Build history of the part. All positions in model axes, mm. A direction names the side the tool comes from. Give positions to 0.01 mm unless a question says otherwise; leave off trailing zeros. Write each loop counter-clockwise with the first axis right and the second up, starting at its lowest first coordinate (ties: lowest second). Pieces come first, ordered by that corner, then holes. Notation, with made-up numbers: (25, 58.25) -> (72, 58.25) arc R21 ccw to (72, 89.25) -> close; hole circle Ø8 at (42.25, 78.5). An arc over 180 degrees is marked (long way). Put each result on its own line as item: value.
from build123d import *

# Parameters (mm, degrees)
SKETCH_1_W                         = 406.5
SKETCH_1_H                         = 22
SM_BASE_FLANGE_1_DEPTH             = 2
SM_EDGE_FLANGE_1_STRIP_W           = 10
SM_EDGE_FLANGE_1_STRIP_H           = 2
SM_EDGE_FLANGE_1_STRIP_CUT_DEPTH   = 406.5
SM_EDGE_FLANGE_1_STRIP_2_W         = 10
SM_EDGE_FLANGE_1_STRIP_2_H         = 2
SM_EDGE_FLANGE_1_STRIP_CUT_2_DEPTH = 406.5
SM_EDGE_FLANGE_1_DEPTH             = 406.5
SM_EDGE_FLANGE_1_BEND_DEPTH        = 406.5
SM_EDGE_FLANGE_2_STRIP_W           = 10
SM_EDGE_FLANGE_2_STRIP_H           = 2
SM_EDGE_FLANGE_2_STRIP_CUT_DEPTH   = 16
SM_EDGE_FLANGE_2_STRIP_2_W         = 10
SM_EDGE_FLANGE_2_STRIP_2_H         = 2
SM_EDGE_FLANGE_2_STRIP_CUT_2_DEPTH = 16
SM_EDGE_FLANGE_2_DEPTH             = 16
SM_EDGE_FLANGE_2_BEND_DEPTH        = 16
SKETCH_18_W                        = 9
SKETCH_18_H                        = 9
CUT_EXTRUDE_1_DEPTH                = 10
PATTERN_LINEAR_1_COUNT             = 19
PATTERN_LINEAR_1_PITCH             = 20
FILLET_1_R                         = 5
SKETCH_19_R                        = 3.5
CUT_EXTRUDE_2_DEPTH                = 408.140332072


# Sheet-metal steps are written as plain solids
with BuildPart() as part:
    # Sketch 1 → 基体-法兰1 (new body)
    with BuildSketch(Plane.XY):
        Rectangle(SKETCH_1_W, SKETCH_1_H)
    extrude(amount=-SM_BASE_FLANGE_1_DEPTH)

    # 边线-法兰1 strip (across the edge) → 边线-法兰1 strip cut (cut)
    with BuildSketch(Plane(origin=(203.25, -11, -2), x_dir=(0, 1, 0), z_dir=(-1, 0, 0))):
        with Locations((-2, -1)):
            Rectangle(SM_EDGE_FLANGE_1_STRIP_W, SM_EDGE_FLANGE_1_STRIP_H)
    extrude(amount=SM_EDGE_FLANGE_1_STRIP_CUT_DEPTH, mode=Mode.SUBTRACT)

    # 边线-法兰1 strip 2 (across the edge) → 边线-法兰1 strip cut 2 (cut)
    with BuildSketch(Plane(origin=(-203.25, 11, -2), x_dir=(0, -1, 0), z_dir=(1, 0, 0))):
        with Locations((-2, -1)):
            Rectangle(SM_EDGE_FLANGE_1_STRIP_2_W, SM_EDGE_FLANGE_1_STRIP_2_H)
    extrude(amount=SM_EDGE_FLANGE_1_STRIP_CUT_2_DEPTH, mode=Mode.SUBTRACT)

    # 边线-法兰1 section (across the edge) → 边线-法兰1 (add)
    with BuildSketch(Plane(origin=(203.25, -11, -2), x_dir=(0, 1, 0), z_dir=(-1, 0, 0))):
        with BuildLine():
            Line((0, 1), (0, 8))
            Line((0, 8), (2, 8))
            Line((2, 8), (2, 1))
            ThreePointArc((2, 1), (2.292893219, 0.292893219), (3, 0))
            Line((3, 0), (3, -2))
            ThreePointArc((3, -2), (0.878679656, -1.121320344), (0, 1))
        make_face()
    extrude(amount=SM_EDGE_FLANGE_1_DEPTH)

    # 边线-法兰1 section 2 (across the edge) → 边线-法兰1 bend (add)
    with BuildSketch(Plane(origin=(-203.25, 11, -2), x_dir=(0, -1, 0), z_dir=(1, 0, 0))):
        with BuildLine():
            Line((0, 1), (0, 8))
            Line((0, 8), (2, 8))
            Line((2, 8), (2, 1))
            ThreePointArc((2, 1), (2.292893219, 0.292893219), (3, 0))
            Line((3, 0), (3, -2))
            ThreePointArc((3, -2), (0.878679656, -1.121320344), (0, 1))
        make_face()
    extrude(amount=SM_EDGE_FLANGE_1_BEND_DEPTH)

    # 边线-法兰2 strip (across the edge) → 边线-法兰2 strip cut (cut)
    with BuildSketch(Plane(origin=(-203.25, -8, -2), x_dir=(1, 0, 0), z_dir=(0, 1, 0))):
        with Locations((-2, -1)):
            Rectangle(SM_EDGE_FLANGE_2_STRIP_W, SM_EDGE_FLANGE_2_STRIP_H)
    extrude(amount=SM_EDGE_FLANGE_2_STRIP_CUT_DEPTH, mode=Mode.SUBTRACT)

    # 边线-法兰2 strip 2 (across the edge) → 边线-法兰2 strip cut 2 (cut)
    with BuildSketch(Plane(origin=(203.25, 8, -2), x_dir=(-1, 0, 0), z_dir=(0, -1, 0))):
        with Locations((-2, -1)):
            Rectangle(SM_EDGE_FLANGE_2_STRIP_2_W, SM_EDGE_FLANGE_2_STRIP_2_H)
    extrude(amount=SM_EDGE_FLANGE_2_STRIP_CUT_2_DEPTH, mode=Mode.SUBTRACT)

    # 边线-法兰2 section (across the edge) → 边线-法兰2 (add)
    with BuildSketch(Plane(origin=(-203.25, -8, -2), x_dir=(1, 0, 0), z_dir=(0, 1, 0))):
        with BuildLine():
            Line((0, 1), (0, 18))
            Line((0, 18), (2, 18))
            Line((2, 18), (2, 1))
            ThreePointArc((2, 1), (2.292893219, 0.292893219), (3, 0))
            Line((3, 0), (3, -2))
            ThreePointArc((3, -2), (0.878679656, -1.121320344), (0, 1))
        make_face()
    extrude(amount=SM_EDGE_FLANGE_2_DEPTH)

    # 边线-法兰2 section 2 (across the edge) → 边线-法兰2 bend (add)
    with BuildSketch(Plane(origin=(203.25, 8, -2), x_dir=(-1, 0, 0), z_dir=(0, -1, 0))):
        with BuildLine():
            Line((0, 1), (0, 18))
            Line((0, 18), (2, 18))
            Line((2, 18), (2, 1))
            ThreePointArc((2, 1), (2.292893219, 0.292893219), (3, 0))
            Line((3, 0), (3, -2))
            ThreePointArc((3, -2), (0.878679656, -1.121320344), (0, 1))
        make_face()
    extrude(amount=SM_EDGE_FLANGE_2_BEND_DEPTH)

    # 草图18 → 切除-拉伸1 (cut)
    with BuildSketch(Plane.XY):
        with Locations((-179.25, 1)):
            Rectangle(SKETCH_18_W, SKETCH_18_H)
    cut_extrude_1 = extrude(amount=-CUT_EXTRUDE_1_DEPTH, mode=Mode.SUBTRACT)

    # 阵列(线性)1: 切除-拉伸1 ×19
    with Locations(*[(i * PATTERN_LINEAR_1_PITCH, 0, 0) for i in range(1, PATTERN_LINEAR_1_COUNT)]):
        add(cut_extrude_1, mode=Mode.SUBTRACT)

    # 圆角1
    fillet_1_edges = [part.edges().sort_by_distance(p)[0] for p in [
        (-202.25, -8, -20),
        (-202.25, 8, -20),
        (202.25, 8, -20),
        (202.25, -8, -20),
    ]]
    fillet(fillet_1_edges, radius=FILLET_1_R)

    # 草图19 → 切除-拉伸2 (cut, through all)
    with BuildSketch(Plane(origin=(203.25, 0, 0), x_dir=(0, 0, -1), z_dir=(1, 0, 0))):
        with Locations((14, 0)):
            Circle(SKETCH_19_R)
    extrude(amount=-CUT_EXTRUDE_2_DEPTH, mode=Mode.SUBTRACT)


solid = part.part
1) Tool access for faces 4 (the flat face through (201.25, 0, -10)), 5 (the flat face through (3, -9, -7)), 6 (the flat face through (42, -5, 0)): list every direction of +Z, -Z, +X, -X, +Y, -Y with a clear straight run to the whole face (end or side of a thin tool).
Filled sheet:
face 4: -Z
face 5: -Z, +X, -X
face 6: +Z, +X, -X, +Y, -Y
2) Pull direction Y, two halves, no side cores. Call faces 1 (the flat face through (42, -5, -2)), 2 (the flat face through (3, -11, -6)), 3 (the flat face through (203.25, 0, -9)): released by +Y, released by -Y, zero draft, split by the parting line, or undercut.
Filled sheet:
face 1: undercut
face 2: released by -Y
face 3: zero draft
3) Wall check: L1, parallel to Y at x = 202.75, z = -14; L2, parallel to X at y = 3.75, z = -3; L3, parallel to Y at x = -187, z = -6.25. Give the ranges that are in metal, low to high.
Filled sheet:
L1: -8 to -3.5, 3.5 to 8
L2: -203.25 to -201.25, 201.25 to 203.25
L3: -11 to -9, 9 to 11
4) Slice it at A-A (x = -150.5). Write the cut outline in (y, z).
Filled sheet:
outline: (-11, -10) -> (-9, -10) -> (-9, -3) arc R1 cw to (-8, -2) -> (8, -2) arc R1 cw to (9, -3) -> (9, -10) -> (11, -10) -> (11, -3) arc R3 ccw to (8, 0) -> (-8, 0) arc R3 ccw to (-11, -3) -> close
5) Pin check, flat tips, straight feed: pin 1 (2 mm diameter, centred on x = -21, z = -1, fed in from +Y); pin 2 (0.9 mm diameter, centred on x = -202, z = -10.5, fed in from -Y); pin 3 (1 mm diameter, centred on x = 120.5, z = -1, fed in from -Y); pin 4 (12 mm diameter, centred on x = 33.5, z = -16.5, fed in from +Y). Stop position of each tip, or through.
Filled sheet:
pin 1: y = 10.83
pin 2: y = -8
pin 3: y = -10.6
pin 4: through
